```python
from build123d import *

# Parameters (mm, degrees)
SKETCH1_R           = 31.75
BOSS_EXTRUDE1_DEPTH = 9.525
BOSS_EXTRUDE2_DEPTH = 19.05
SKETCH3_R           = 1.143
CUT_EXTRUDE1_DEPTH  = 43.730618225
SKETCH4_W           = 11.567255286
SKETCH4_H           = 3.936355762
CUT_EXTRUDE2_DEPTH  = 93.234251534


with BuildPart() as part:
    # Sketch1 → Boss-Extrude1 (new body)
    with BuildSketch(Plane.XY):
        with BuildLine():
            Line((-5.900618225, 36.354251534), (5.900618225, 36.354251534))
            ThreePointArc((5.900618225, 36.354251534), (0, -36.83), (-5.900618225, 36.354251534))
        make_face()
        Circle(SKETCH1_R, mode=Mode.SUBTRACT)
    extrude(amount=BOSS_EXTRUDE1_DEPTH)

    # Sketch2 → Boss-Extrude2 (add)
    with BuildSketch(Plane(origin=(0, 36.354251534, 0), x_dir=(1, 0, 0), z_dir=(0, 1, 0))):
        with BuildLine():
            Line((-3.067713808, -9.525), (3.067713808, -9.525))
            ThreePointArc((3.067713808, -9.525), (0, 0.902504348), (-3.067713808, -9.525))
        make_face()
    extrude(amount=BOSS_EXTRUDE2_DEPTH)

    # Sketch3 → Cut-Extrude1 (cut, through all)
    with BuildSketch(Plane(origin=(5.900618225, 0, 0), x_dir=(0, 0, -1), z_dir=(1, 0, 0))):
        with Locations((-4.546893104, 45.879251534)):
            Circle(SKETCH3_R)
    extrude(amount=-CUT_EXTRUDE1_DEPTH, mode=Mode.SUBTRACT)

    # Sketch4 → Cut-Extrude2 (cut, through all)
    with BuildSketch(Plane(origin=(0, 55.404251534, 0), x_dir=(1, 0, 0), z_dir=(0, 1, 0))):
        with Locations((-0.26002139, -11.608026225)):
            Rectangle(SKETCH4_W, SKETCH4_H)
    extrude(amount=-CUT_EXTRUDE2_DEPTH, mode=Mode.SUBTRACT)


solid = part.part
```
CAD build for the part. Positions are in the model's coordinates, mm. A direction names the side the tool comes from. Give positions to 0.01 mm unless a question says otherwise; leave off trailing zeros. Loops run counter-clockwise (first coordinate to the right, second up) from the corner with the lowest first, then second, coordinate; pieces in that order, holes last. Notation, with made-up numbers: (56, -9) - (109, -9) arc R26 ccw to (109, 23) - close; hole circle Ø4 at (41, 41.25). An arc over 180 degrees is marked (long way). Put each result on its own line as item: value.
Q1. Slice it at B-B (x = -17). Give the cut face in (y, z) (3 decimals), plus the area to 3 significant figures.
Filled in:
outline: (-32.672, 0) - (-26.815, 0) - (-26.815, 9.525) - (-32.672, 9.525) - close; (26.815, 0) - (32.672, 0) - (32.672, 9.525) - (26.815, 9.525) - close
area: 112 mm²
Q2. Slice it at C-C (x = 0). Give the number of separate pieces and of enclosed holes in the cut face, plus the area to 3 significant figures.
Filled in:
separate pieces: 2
enclosed holes: 1
area: 287 mm²
Q3. Flat gauge pins, fed straight in: pin 1 (3 mm diameter, centred on y = 29, z = 6.5, fed in from +X); pin 2 (1 mm diameter, centred on y = 33, z = 7.5, fed in from +X); pin 3 (1.5 mm diameter, centred on x = 20.5, z = 7, fed in from -Y). Where does each tip first touch, or does it go through?
Filled in:
pin 1: stops at x = 24.5
pin 2: stops at x = 17.33
pin 3: stops at y = -31.09
Q4. Tool access for faces 1 (the face through (0.2, 45.7, -0.9)), 2 (the face through (0.08, 47.01, 4.7)), 3 (the face through (-5.75, 36.354, 5.8)): list every direction of +Z, -Z, +X, -X, +Y, -Y with a clear straight run to the whole face (end or side of a thin tool).
Filled in:
face 1: +Y
face 2: +X, -X
face 3: -X, +Y
Q5. Mould opens along X. For faces 4 (the face through (1.5, -36.8, 4.7)), 5 (the face through (-6.883, -30.995, 4.696)), 6 (the face through (-14, 30, 9.525)) say: pulls with the +X half, pulls with the -X half, needs draft (parallel to the pull), parting line crosses it, or undercut.
Filled in:
face 4: parting line crosses it
face 5: undercut
face 6: needs draft
Q6. Slice it at A-A (y = 0). Give the cut face in (x, z) (3 decimals), plus the area to 3 significant figures.
Filled in:
outline: (-36.83, 0) - (-31.75, 0) - (-31.75, 9.525) - (-36.83, 9.525) - close; (31.75, 0) - (36.83, 0) - (36.83, 9.525) - (31.75, 9.525) - close
area: 96.8 mm²
Q7. Slice it at D-D (z = 1.25). Give the cut face in (x, y).
Filled in:
outline: (-5.9, 36.35) arc R36.83 ccw (long way) to (5.9, 36.35) - (4.44, 36.35) - (4.44, 55.4) - (-4.44, 55.4) - (-4.44, 36.35) - close; hole circle Ø63.5 at (0, 0)
Q8. Probe line 1 along Z through (x, y) = (18, -29.5) (3 decimals); line 2 along Y through (x, z) = (26.5, 7); line 3 along Y through (x, z) = (0, 5.25). List the from-to ranges inside material, lowest first.
Filled in:
line 1: z = 0 to 9.525
line 2: y = -25.58 to -17.49, 17.49 to 25.58
line 3: y = -36.83 to -31.75, 31.75 to 44.98, 46.78 to 55.4
